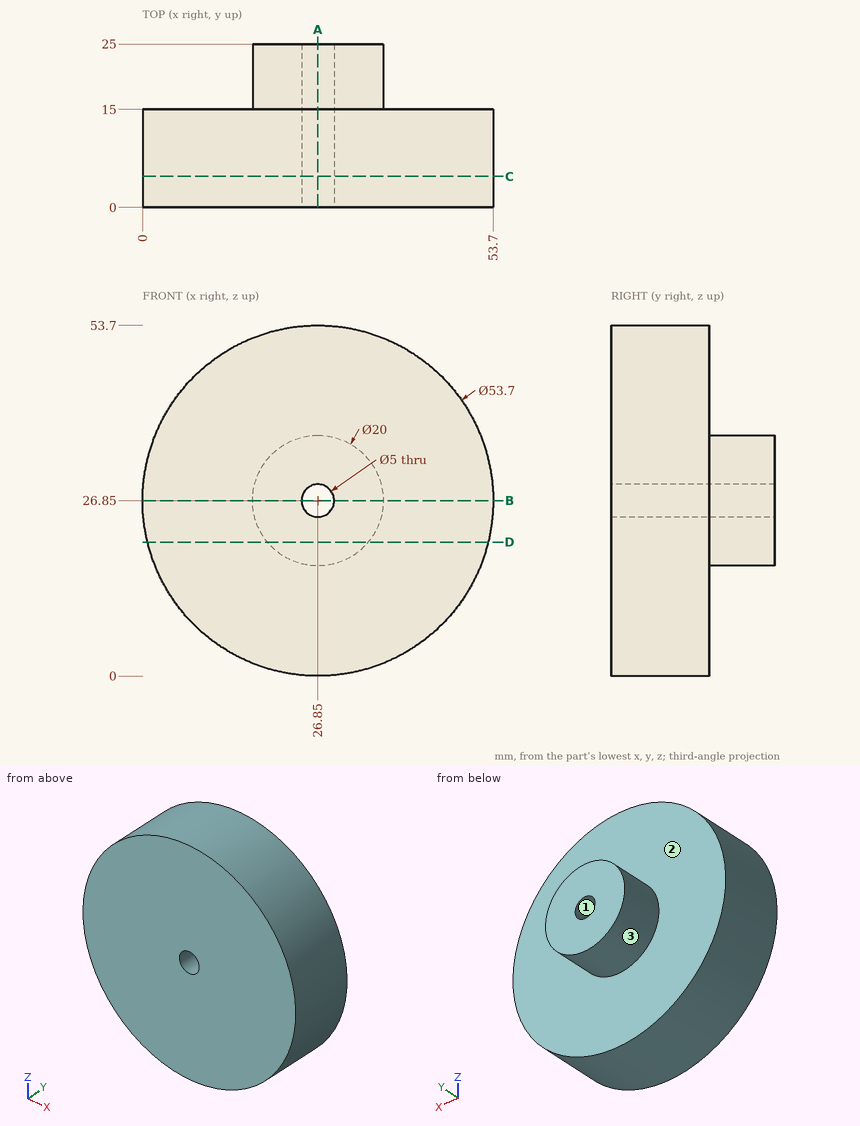
The drawing under review shows one solid part. Ordinate dimensions are in mm from its lowest x, y, z. Give positions to 0.01 mm unless a question says otherwise; leave off trailing zeros. Loops run counter-clockwise (first coordinate to the right, second up) from the corner with the lowest first, then second, coordinate; pieces in that order, holes last. Notation, with made-up numbers: M -17,-18.5 L -11,-18.5 A32 ccw -11,12.5 Z; hole C 40.25,24.25 d5. An arc over 180 degrees is marked long. One line per item, written item: value. Start each with the question number.
Q1. For L1, parallel to X at y = 5.5, z = 26.85; L2, parallel to X at y = 16.5, z = 27; L3, parallel to Y at x = 9, z = 42.5, list the stretches that pass through material, from the lowest coordinate up.
Q2. Clearance check with flat-ended pins moving along their axes: pin 1 Ø5 at (y, z) = (10.5, 25) entering from -X; pin 2 Ø6 at (x, y) = (9.5, 10) entering from -Z; pin 3 Ø1.5 at (y, z) = (20, 32) entering from +X; pin 4 Ø4 at (x, z) = (26.85, 26.85) entering from +Y. State where each tip first meets the part, or that it passes through.
Q3. Add section A-A (x = 26.85). Give the boundary of the cut face in (y, z).
Q4. Add section C-C (y = 4.75). Give the boundary of the cut face in (x, z).
Q5. Add section B-B (z = 26.85). Give the boundary of the cut face in (x, y), and give its area (4 significant figures).
Q6. Draft analysis for pull direction X (two halves, no side actions). For the marked faces 1, 2 and 3, state which applies: released by +X, released by -X, zero draft, split by the parting line, or undercut.
Q7. Add section D-D (z = 20.5). Give the boundary of the cut face in (x, y).
Reply:
1. L1: 0 to 24.35, 29.35 to 53.7
1. L2: 16.85 to 24.35, 29.35 to 36.85
1. L3: 0 to 15
2. pin 1: x = 0
2. pin 2: z = 4.16
2. pin 3: x = 35.83
2. pin 4: through
3. outline: M 0,0 L 15,0 L 15,16.85 L 25,16.85 L 25,24.35 L 0,24.35 Z; M 0,29.35 L 25,29.35 L 25,36.85 L 15,36.85 L 15,53.7 L 0,53.7 Z
4. outline: C 26.85,26.85 d53.7; hole C 26.85,26.85 d5
5. outline: M 0,0 L 24.35,0 L 24.35,25 L 16.85,25 L 16.85,15 L 0,15 Z; M 29.35,0 L 53.7,0 L 53.7,15 L 36.85,15 L 36.85,25 L 29.35,25 Z
5. area: 880.5 mm²
6. face 1: undercut
6. face 2: zero draft
6. face 3: split by the parting line
7. outline: M 0.76,0 L 52.94,0 L 52.94,15 L 34.58,15 L 34.58,25 L 19.12,25 L 19.12,15 L 0.76,15 Z
